For this review, take the finished solid that the model builds, in its own axes (mm). Face numbers are marked on the shaded views. Round coordinates to 2 decimals unless told otherwise and drop trailing zeros. Loops run counter-clockwise (first coordinate to the right, second up) from the corner with the lowest first, then second, coordinate; pieces in that order, holes last.
1. Consider section B-B on y = 60. State the section outline as (x, z) points (1 decimal).
2. Clearance check with flat-ended pins moving along their axes: pin 1 Ø4.5 at (x, z) = (1, 0) entering from -Y; pin 2 Ø1.5 at (y, z) = (20.5, 1) entering from +X; pin 3 Ø5 at (y, z) = (68, 3.5) entering from -X; pin 4 Ø1.5 at (y, z) = (65, 4) entering from -X. State where each tip first meets the part, or that it passes through.
3. Consider section A-A on y = 24. State the section outline as (x, z) points (1 decimal), then the cut area to 3 significant figures.
4. To check wall thickness, follow line 1 along X through (y, z) = (42, 0); line 2 along Z through (x, y) = (-0.75, 53); line 3 along Z through (x, y) = (-0.75, 24). State the ranges of each line that lie inside material, in increasing order.
5. Draft analysis for pull direction Y (two halves, no side actions). For the marked faces 1 and 2, state which applies: released by +Y, released by -Y, zero draft, split by the parting line, or undercut.
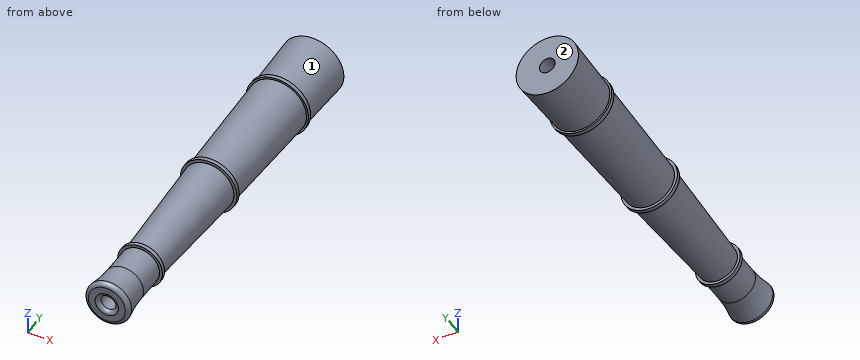
from build123d import *

# Parameters (mm, degrees)
F2_R = 0.79375


with BuildPart() as f1:
    # F0 (on Right) → F1 (revolve)
    with BuildSketch(Plane.YZ):
        with BuildLine():
            Line((0, 1.5875), (12.303125, 1.5875))
            Line((12.303125, 1.5875), (12.303125, 3.96875))
            Line((12.303125, 3.96875), (6.35, 3.96875))
            ThreePointArc((6.35, 3.96875), (3.1502914561, 4.1679566492), (0, 4.7625))
            Line((0, 4.7625), (0, 1.5875))
        make_face()
        Polygon((12.303125, 1.5875), (13.096875, 1.5875), (13.096875, 3.9873535156), (12.7, 3.96875), (12.303125, 3.96875), align=None)
        Polygon((12.7, 3.96875), (13.096875, 3.9873535156), (13.096875, 4.5640625), (12.303125, 4.5640625), (12.303125, 3.96875), align=None)
        Polygon((13.096875, 1.5875), (37.703125, 1.5875), (37.703125, 5.1407714844), (13.096875, 3.9873535156), align=None)
        Polygon((37.703125, 1.5875), (38.496875, 1.5875), (38.496875, 5.1717773437), (38.1, 5.159375), (37.703125, 5.1407714844), align=None)
        Polygon((38.1, 5.159375), (38.496875, 5.1717773437), (38.496875, 5.7546875), (37.703125, 5.7546875), (37.703125, 5.1407714844), align=None)
        Polygon((38.496875, 1.5875), (63.103125, 1.5875), (63.103125, 5.9407226563), (38.496875, 5.1717773437), align=None)
        Polygon((63.896875, 1.5875), (76.2, 1.5875), (76.2, 6.35), (63.896875, 5.9655273437), align=None)
        Polygon((63.103125, 1.5875), (63.896875, 1.5875), (63.896875, 5.9655273437), (63.5, 5.953125), (63.103125, 5.9407226563), align=None)
        Polygon((63.5, 5.953125), (63.896875, 5.9655273437), (63.896875, 6.35), (63.103125, 6.35), (63.103125, 5.9407226563), align=None)
    revolve(axis=Axis((0, 38.1, 0), (0, 1, 0)))

    # F2
    f2_edges = [f1.edges().sort_by_distance(p)[0] for p in [
        (0, 0, -4.7625),
        (0, 0, -1.5875),
    ]]
    fillet(f2_edges, radius=F2_R)


solid = f1.part
Resolved:
1. outline: circle Ø11.7 at (0, 0); hole circle Ø3.2 at (0, 0)
2. pin 1: stops at y = 0
2. pin 2: stops at x = 4.34
2. pin 3: stops at x = -6.02
2. pin 4: stops at x = -5.04
3. outline: circle Ø9 at (0, 0); hole circle Ø3.2 at (0, 0)
3. area: 55.7 mm2
4. line 1: x = -5.28 to -1.59, 1.59 to 5.28
4. line 2: z = -5.57 to -1.4, 1.4 to 5.57
4. line 3: z = -4.44 to -1.4, 1.4 to 4.44
5. face 1: undercut
5. face 2: released by +Y
